Can you work these out from the model? Positions are in its coordinate system, mm. A direction names the side the tool comes from. Coordinates: 2 decimals unless noted, no trailing zeros. Order: outer loops, then holes, each group sorted by start corner. A loop starts at its lowest first (then second) coordinate and runs counter-clockwise, first axis right, second up. Notation, with made-up numbers: (-29, 51) -> (25, 51) arc R8 ccw to (25, 59) -> close; hole circle Ø9 at (32.5, 82). An arc over 180 degrees is marked (long way). Write item = value, one per line. Start each with the question number.
from build123d import *

# Parameters (mm, degrees)
SKETCH1_R               = 1.25
BOSS_EXTRUDE1_DEPTH     = 42.5
SKETCH2_OUTSIDE_W       = 13.03
SKETCH2_OUTSIDE_H       = 13.03
SKETCH2_OUTSIDE_R       = 1
CUT_EXTRUDE1_DEPTH      = 3.5
SKETCH3_OUTSIDE_W       = 13.03
SKETCH3_OUTSIDE_H       = 13.03
SKETCH3_OUTSIDE_R       = 0.7
CUT_EXTRUDE2_DEPTH      = 2
CHAMFER1_SIZE           = 0.2
SKETCH4_W               = 0.8
SKETCH4_H               = 4
CUT_EXTRUDE3_DEPTH      = 2.25
CUT_EXTRUDE3_DEPTH_BACK = 2.25
LPATTERN1_COUNT         = 2
LPATTERN1_PITCH         = 3.95


with BuildPart() as part:
    # Sketch1 → Boss-Extrude1 (new body)
    with BuildSketch(Plane(origin=(0, 0, 0), x_dir=(1, 0, 0), z_dir=(0, 1, 0))):
        Circle(SKETCH1_R)
    extrude(amount=BOSS_EXTRUDE1_DEPTH)

    # Sketch2 outside → Cut-Extrude1 (cut)
    with BuildSketch(Plane(origin=(0, 42.5, 0), x_dir=(1, 0, 0), z_dir=(0, 1, 0))):
        Rectangle(SKETCH2_OUTSIDE_W, SKETCH2_OUTSIDE_H)
        Circle(SKETCH2_OUTSIDE_R, mode=Mode.SUBTRACT)
    extrude(amount=-CUT_EXTRUDE1_DEPTH, mode=Mode.SUBTRACT)

    # Sketch3 outside → Cut-Extrude2 (cut)
    with BuildSketch(Plane(origin=(0, 42.5, 0), x_dir=(1, 0, 0), z_dir=(0, 1, 0))):
        Rectangle(SKETCH3_OUTSIDE_W, SKETCH3_OUTSIDE_H)
        Circle(SKETCH3_OUTSIDE_R, mode=Mode.SUBTRACT)
    extrude(amount=-CUT_EXTRUDE2_DEPTH, mode=Mode.SUBTRACT)

    # Chamfer1
    chamfer1_edges = [part.edges().sort_by_distance(p)[0] for p in [
        (-0.7, 42.5, 0),
    ]]
    chamfer(chamfer1_edges, length=CHAMFER1_SIZE)

    # Sketch4 → Cut-Extrude3 (cut, two sides)
    with BuildSketch(Plane(origin=(0, 0, 0), x_dir=(0, 0, -1), z_dir=(1, 0, 0))) as cut_extrude3_sk:
        with Locations((0.85, 4.5)):
            Rectangle(SKETCH4_W, SKETCH4_H)
        with Locations((-0.85, 4.5)):
            Rectangle(SKETCH4_W, SKETCH4_H)
    extrude(amount=CUT_EXTRUDE3_DEPTH, mode=Mode.SUBTRACT)
    extrude(cut_extrude3_sk.sketch, amount=-CUT_EXTRUDE3_DEPTH_BACK, mode=Mode.SUBTRACT)

    # Sketch5 → Cut-Revolve2 (revolve, cut)
    with BuildSketch(Plane.XY):
        Polygon((1.25, 32.123358295), (0.27, 30.2), (1.25, 30.2), align=None)
    cut_revolve2 = revolve(axis=Axis((0.27, 30.2, 0), (1, 0, 0)), mode=Mode.SUBTRACT)

    # LPattern1: Cut-Revolve2 ×2
    with Locations(*[(0, -i * LPATTERN1_PITCH, 0) for i in range(1, LPATTERN1_COUNT)]):
        add(cut_revolve2, mode=Mode.SUBTRACT)


solid = part.part
(1) For P1, Ø0.6, axis at x = 0.5, z = -1, coming from the -Y side; P2, Ø0.7, axis at x = 0, y = 4, coming from the +Z side; P3, Ø1.2, axis at x = 0.5, y = 4, coming from the -Z side, each with a flat end and sliding along its axis, tell me the tip position at first contact or that it passes through.
(2) For faces 1 (the face through (0, 40, 1)), 2 (the face through (0, 0, 0)), 3 (the face through (0, 4, 0.45)), which set-ups out of +Z, -Z, +X, -X, +Y, -Y let a thin tool reach every point of the face, with its end or its side?
(3) If I drill on L1, parallel to Y at x = -0.6, z = 0.75; L2, parallel to Y at x = 0.5, z = 0.15; L3, parallel to Y at x = 1, z = -0.3, over which ranges is the centre line in solid material (lowest first)? Write a range as from..to.
(4) Thinking about a two-plate mould opening in Y: for faces 4 (the face through (0, 42.5, 0)), 5 (the face through (0, 4, -0.45)), 6 (the face through (0.32, 26.34, -0.04)), 7 (the face through (-1.25, 19.23, -0.05)), which applies, +Y half, -Y half, draft (parallel to the pull), parting line (faces both ways), or undercut?
(5) Imagine slicing it at A-A (y = 33.5). Write out the boundary of the cut face in (x, z).
Result set:
q1.P1 = 0
q1.P2 = 0.45
q1.P3 = -0.45
q2.face_1 = +Y
q2.face_2 = +Z, -Z, +X, -X, -Y
q2.face_3 = +Z, +X, -X
q3.L1 = 0..2.5, 6.5..40.5
q3.L2 = 0..25.82, 26.68..29.77, 30.63..42.48
q3.L3 = 0..24.85, 27.65..28.8, 31.6..39
q4.face_4 = +Y half
q4.face_5 = undercut
q4.face_6 = undercut
q4.face_7 = draft
q5.outline = circle Ø2.5 at (0, 0)
